Geometry: final body of the model. Coordinates: model frame, mm. A direction names the side the tool comes from. Coordinates: 2 decimals unless noted, no trailing zeros. Order: outer loops, then holes, each group sorted by start corner. A loop starts at its lowest first (then second) coordinate and runs counter-clockwise, first axis right, second up. Notation, with made-up numbers: M 58,41.5 L 99,41.5 A9 cw 99,52.5 Z; hole C 80.25,-28 d2. An arc over 180 degrees is marked long. One line per question, with ' | ' between items.
from build123d import *

# Parameters (mm, degrees)
SKETCH1_R               = 12.446
SKETCH1_R_2             = 4.318
BOSS_EXTRUDE1_DEPTH     = 22.86
SKETCH2_R               = 3.175
CUT_EXTRUDE1_DEPTH      = 13.446
SKETCH4_R               = 25.4
SKETCH4_R_2             = 5.715
CUT_EXTRUDE3_DEPTH      = 15.24
SKETCH7_R               = 1.27
CUT_EXTRUDE4_DEPTH      = 5.334
CUT_EXTRUDE4_DEPTH_BACK = 1.5080001
SKETCH8_R               = 5.715
SKETCH8_R_2             = 4.318
BOSS_EXTRUDE2_DEPTH     = 1.524
CHAMFER1_SIZE           = 0.508
SKETCH9_R               = 23.611709968
SKETCH9_W               = 20.32
SKETCH9_H               = 32.6206423
CUT_EXTRUDE5_DEPTH      = 13.97


with BuildPart() as part:
    # Sketch1 → Boss-Extrude1 (new body)
    with BuildSketch(Plane(origin=(0, 0, 0), x_dir=(0, 0, -1), z_dir=(1, 0, 0))):
        Circle(SKETCH1_R)
        Circle(SKETCH1_R_2, mode=Mode.SUBTRACT)
    extrude(amount=BOSS_EXTRUDE1_DEPTH)

    # Sketch2 → Cut-Extrude1 (cut, symmetric)
    with BuildSketch(Plane.XY):
        with Locations((19.05, 8.382)):
            Circle(SKETCH2_R)
    cut_extrude1 = extrude(amount=CUT_EXTRUDE1_DEPTH, both=True, mode=Mode.SUBTRACT)

    # Mirror1: Cut-Extrude1 across plane
    add(cut_extrude1.mirror(Plane.ZX), mode=Mode.SUBTRACT)

    # Sketch4 → Cut-Extrude3 (cut)
    with BuildSketch(Plane.ZY):
        Circle(SKETCH4_R)
        Circle(SKETCH4_R_2, mode=Mode.SUBTRACT)
    extrude(amount=-CUT_EXTRUDE3_DEPTH, mode=Mode.SUBTRACT)

    # Sketch7 → Cut-Extrude4 (cut, two sides)
    with BuildSketch(Plane(origin=(0, 0, 11.938), x_dir=(1, 0, 0), z_dir=(0, 0, -1))) as cut_extrude4_sk:
        with Locations((19.812, 0)):
            Circle(SKETCH7_R)
    extrude(amount=CUT_EXTRUDE4_DEPTH, mode=Mode.SUBTRACT)
    extrude(cut_extrude4_sk.sketch, amount=-CUT_EXTRUDE4_DEPTH_BACK, mode=Mode.SUBTRACT)

    # Sketch8 → Boss-Extrude2 (add)
    with BuildSketch(Plane.ZY):
        Circle(SKETCH8_R)
        Circle(SKETCH8_R_2, mode=Mode.SUBTRACT)
    extrude(amount=BOSS_EXTRUDE2_DEPTH)

    # Chamfer1
    chamfer1_edges = [part.edges().sort_by_distance(p)[0] for p in [
        (15.24, 0, 12.446),
        (-1.524, 0, -5.715),
        (22.86, 0, 12.446),
    ]]
    chamfer(chamfer1_edges, length=CHAMFER1_SIZE)

    # Sketch9 → Cut-Extrude5 (cut)
    with BuildSketch(Plane.ZY.offset(-15.24)):
        Circle(SKETCH9_R)
        Rectangle(SKETCH9_W, SKETCH9_H, mode=Mode.SUBTRACT)
    extrude(amount=-CUT_EXTRUDE5_DEPTH, mode=Mode.SUBTRACT)


solid = part.part
1. Section B-B, the plane z = 0. Output: boundary loops of the cut face in (x, y) (3 decimals), and give its area (3 significant figures).
Response values:
outline: M -1.524,-5.207 L -1.016,-5.715 L 15.24,-5.715 L 15.24,-11.938 L 15.748,-12.446 L 22.352,-12.446 L 22.86,-11.938 L 22.86,-4.318 L -1.524,-4.318 Z; M -1.524,4.318 L 22.86,4.318 L 22.86,11.938 L 22.352,12.446 L 15.748,12.446 L 15.24,11.938 L 15.24,5.715 L -1.016,5.715 L -1.524,5.207 Z; hole C 19.05,-8.382 d6.35; hole C 19.05,8.382 d6.35 | area: 107 mm^2
2. Draft query along X for faces 1 (the face through (22.722, -12.074, 0.172)), 2 (the face through (18.362, 5.283, 0.142)), 3 (the face through (15.385, -12.081, -0.172)), 4 (the face through (18.543, -0.056, 8.407)). Return one class per face: pulls with the +X half, pulls with the -X half, needs draft (parallel to the pull), parting line crosses it, or undercut.
Response values:
face 1: pulls with the +X half | face 2: undercut | face 3: pulls with the -X half | face 4: undercut
3. Section C-C, the plane x = 19. Output: boundary loops of the cut face in (y, z), and give its area (3 significant figures).
Response values:
outline: M -11.56,-4.62 L -11.56,4.62 A12.45 ccw Z; M -5.21,-10.16 L 5.21,-10.16 L 5.21,10.16 L 0.98,10.16 L 0.98,6.6 L -0.98,6.6 L -0.98,10.16 L -5.21,10.16 Z; M 11.56,-4.62 A12.45 ccw 11.56,4.62 Z; hole C 0,0 d8.64 | area: 157 mm^2
4. Access query for faces 5 (the face through (20, 0, 6.604)), 6 (the face through (15.385, 12.081, 0.172)), 7 (the face through (15.24, 5.5, 2.1)). Directions: +Z, -Z, +X, -X, +Y, -Y. A direction counts if a zero-diameter tool reaches every point of the face in a straight line with its end or side. Return the directions, or none.
Response values:
face 5: +Z | face 6: -X, +Y | face 7: -X
5. Section D-D, the plane z = 2.5. Give the number of separate pieces and of enclosed holes in the cut face, and give its area (3 significant figures).
Response values:
separate pieces: 2 | enclosed holes: 2 | area: 122 mm^2
6. Pin query (flat end, axial travel): P1, Ø1, axis at x = 3, z = 1, coming from the -Y side; P2, Ø1.5, axis at y = 1.5, z = 7.5, coming from the -X side; P3, Ø5, axis at x = 5, y = 0.5, coming from the -Z side (3 decimals). Return the tip coordinate at first contact, or that it passes through.
Response values:
P1: stops at y = -5.69 | P2: stops at x = 15.24 | P3: stops at z = -5.715
7. Section A-A, the plane y = 0. Output: boundary loops of the cut face in (x, z) (3 decimals), and give its area (3 significant figures).
Response values:
outline: M -1.524,-5.207 L -1.016,-5.715 L 15.24,-5.715 L 15.24,-10.16 L 22.86,-10.16 L 22.86,-4.318 L -1.524,-4.318 Z; M -1.524,4.318 L 22.86,4.318 L 22.86,10.16 L 21.082,10.16 L 21.082,6.604 L 18.542,6.604 L 18.542,10.16 L 15.24,10.16 L 15.24,5.715 L -1.016,5.715 L -1.524,5.207 Z | area: 127 mm^2
8. Material intervals for line 1 (Y direction, x = -0.4, z = 0) (3 decimals); line 2 (X direction, y = 0, z = 9.15); line 3 (Z direction, x = 15, y = -1.25), sorted ascending. Write a range as [from, to].
Response values:
line 1: y = [-5.715, -4.318], [4.318, 5.715] | line 2: x = [15.24, 18.54], [21.08, 22.86] | line 3: z = [-5.58, -4.13], [4.13, 5.58]
